Design review of the part shown in the three views and the two pictorial views. Dimensions are in mm from the part's minimum x, y and z. Round coordinates to 2 decimals unless told otherwise and drop trailing zeros. Loops run counter-clockwise (first coordinate to the right, second up) from the corner with the lowest first, then second, coordinate; pieces in that order, holes last. Notation, with made-up numbers: (0.5, -21) -> (11.5, -21) arc R12 cw to (11.5, -11) -> close; hole circle Ø4 at (49, 52). An arc over 180 degrees is marked (long way). Use a Markdown table: item, result. Add a question column.
1) Consider section A-A on z = 78. Give the boundary of the cut face in (x, y) (3 decimals).
2) Wall thickness on probe 1 along X at (y, z) = (2.85, 103) (3 decimals); probe 2 along X at (y, z) = (1.7, 82.5) (3 decimals); probe 3 along Z at (x, y) = (178, 0.4) (3 decimals): over which ranges is each line inside the solid? List them lowest first.
3) Insertion check: pin 1 (1.6 mm diameter, centred on y = 1, z = 16.5, fed in from +X); pin 2 (1.5 mm diameter, centred on x = 87, y = 2.5, fed in from +Z); pin 3 (1 mm diameter, centred on y = 2, z = 104.5, fed in from -X). Each pin has a flat end and moves straight along its axis. Give the tip position at first contact, or say it passes through.
4) Consider section C-C on z = 102. Give the boundary of the cut face in (x, y) (3 decimals), plus the area to 3 significant figures.
5) Consider section D-D on x = 90. Give the boundary of the cut face in (y, z) (3 decimals).
6) Consider section B-B on y = 0.6. Give the boundary of the cut face in (x, z) (3 decimals), plus the area to 3 significant figures.
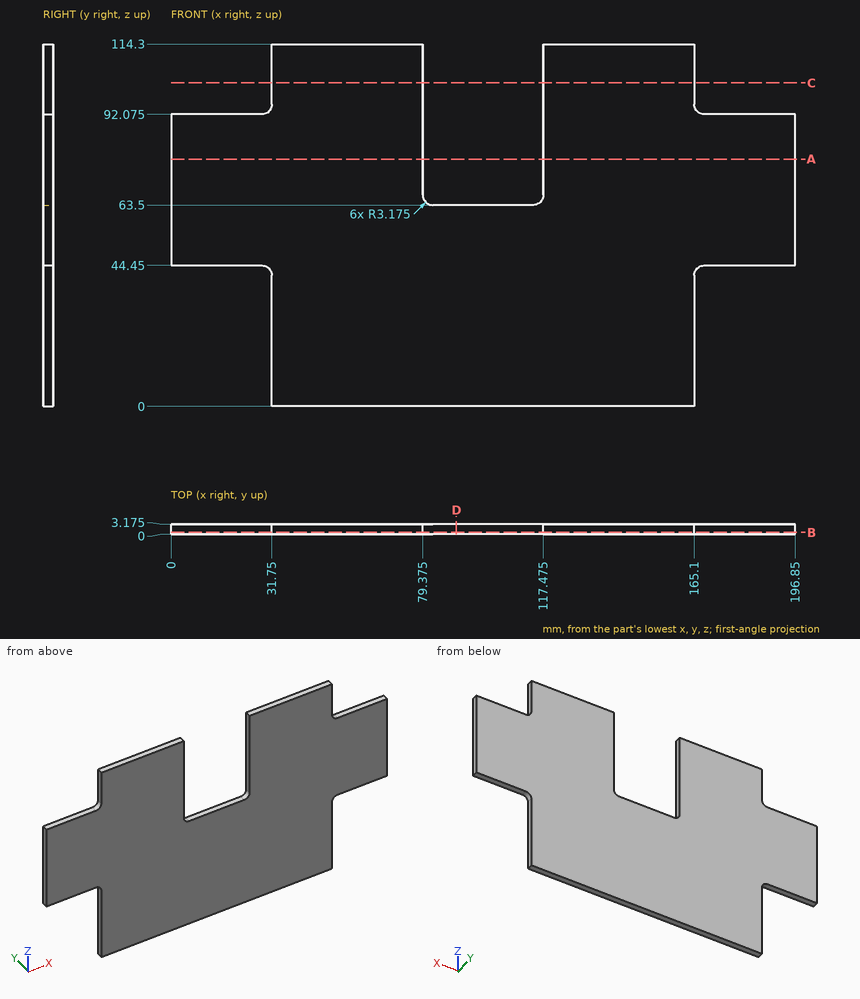
Result set:
| question | item | result |
|---|---|---|
| 1 | outline | (0, 0) -> (79.375, 0) -> (79.375, 3.175) -> (0, 3.175) -> close; (117.475, 0) -> (196.85, 0) -> (196.85, 3.175) -> (117.475, 3.175) -> close |
| 2 | probe 1 | 31.75 to 79.375, 117.475 to 165.1 |
| 2 | probe 2 | 0 to 79.375, 117.475 to 196.85 |
| 2 | probe 3 | 44.45 to 92.075 |
| 3 | pin 1 | x = 165.1 |
| 3 | pin 2 | z = 63.5 |
| 3 | pin 3 | x = 31.75 |
| 4 | outline | (31.75, 0) -> (79.375, 0) -> (79.375, 3.175) -> (31.75, 3.175) -> close; (117.475, 0) -> (165.1, 0) -> (165.1, 3.175) -> (117.475, 3.175) -> close |
| 4 | area | 302 mm2 |
| 5 | outline | (0, 0) -> (3.175, 0) -> (3.175, 63.5) -> (0, 63.5) -> close |
| 6 | outline | (0, 44.45) -> (28.575, 44.45) arc R3.175 cw to (31.75, 41.275) -> (31.75, 0) -> (165.1, 0) -> (165.1, 41.275) arc R3.175 cw to (168.275, 44.45) -> (196.85, 44.45) -> (196.85, 92.075) -> (168.275, 92.075) arc R3.175 cw to (165.1, 95.25) -> (165.1, 114.3) -> (117.475, 114.3) -> (117.475, 66.675) arc R3.175 cw to (114.3, 63.5) -> (82.55, 63.5) arc R3.175 cw to (79.375, 66.675) -> (79.375, 114.3) -> (31.75, 114.3) -> (31.75, 95.25) arc R3.175 cw to (28.575, 92.075) -> (0, 92.075) -> close |
| 6 | area | 16,300 mm2 |
